The model under review builds one solid part; all positions refer to its coordinate system, in mm. A direction names the side the tool comes from. Round coordinates to 2 decimals unless told otherwise and drop trailing zeros. Loops run counter-clockwise (first coordinate to the right, second up) from the corner with the lowest first, then second, coordinate; pieces in that order, holes last. Notation, with made-up numbers: (46.25, 44) -> (67.25, 44) arc R20 cw to (67.25, 73) -> close; hole circle Ø7 at (-3, 11.25). An arc over 180 degrees is marked (long way). Use a Markdown table: item, result. Add a question column.
1) Consider section A-A on y = 3.75. Give the boundary of the cut face in (x, z).
2) Insertion check: pin 1 (1.6 mm diameter, centred on y = 5.715, z = -11.525, fed in from +X); pin 2 (4 mm diameter, centred on x = 8.5, y = 6.5, fed in from -Z). Each pin has a flat end and moves straight along its axis. Give the tip position at first contact, or say it passes through.
3) Wall thickness on probe 1 along X at (y, z) = (6, -9.5); probe 2 along Y at (x, z) = (1.25, -20.5) (3 decimals); probe 3 along Z at (x, y) = (5.75, 5.75): over which ranges is each line inside the solid? List them lowest first.
4) For faces 1 (the flat face through (-11.112, 2, -2)), 2 (the flat face through (8, 6, -14.7)), 3 (the flat face through (-8, 6, -8.35)), 4 (the flat face through (-4.762, 4, -11)), 5 (the flat face through (0, 2, 20.6)), list the 3-axis set-ups (+Z, -Z, +X, -X, +Y, -Y) from which the entire face can be reached by the end or side of a thin tool; tool diameter is ignored.
5) Consider section C-C on z = -4. Give the boundary of the cut face in (x, y) (1 decimal).
6) Mouldability with a two-part tool opening along Y and no side actions: class faces 6 (the flat face through (4.762, 4, -11)), 7 (the flat face through (8, 7.984, -12)), 8 (the cylindrical face through (7.982, 4.826, -11.988)), 9 (the flat face through (0, 0, -3)) as released by +Y, released by -Y, zero draft, split by the parting line, or undercut.
from build123d import *

# Parameters (mm, degrees)
SKETCH1_W             = 22.225
SKETCH1_H             = 46
BOSS_EXTRUDE1_DEPTH   = 3.175
SKETCH2_W             = 6.35
SKETCH2_H             = 6.35
BOSS_EXTRUDE2_DEPTH   = 4.80949
F_1_0MM_DOWEL_HOLE1_D = 2.005


with BuildPart() as part:
    # Sketch1 → Boss-Extrude1 (new body)
    with BuildSketch(Plane(origin=(0, 0, 0), x_dir=(1, 0, 0), z_dir=(0, 1, 0))):
        with Locations((0, 2.4)):
            Rectangle(SKETCH1_W, SKETCH1_H)
    extrude(amount=BOSS_EXTRUDE1_DEPTH)

    # Sketch2 → Boss-Extrude2 (add)
    with BuildSketch(Plane(origin=(0, 3.175, 0), x_dir=(1, 0, 0), z_dir=(0, 1, 0))):
        with Locations((7.9375, 11.525)):
            Rectangle(SKETCH2_W, SKETCH2_H)
    boss_extrude2 = extrude(amount=BOSS_EXTRUDE2_DEPTH)

    # Ø1.0mm Dowel Hole1 (through all)
    with Locations(Plane.ZY.offset(-4.7625)):
        with Locations((-11.525, 5.715)):
            f_1_0mm_dowel_hole1 = Hole(F_1_0MM_DOWEL_HOLE1_D / 2)

    # Mirror1: Boss-Extrude2, Ø1.0mm Dowel Hole1 across plane
    add(boss_extrude2.mirror(Plane.ZY))
    add(f_1_0mm_dowel_hole1.mirror(Plane.ZY), mode=Mode.SUBTRACT)


solid = part.part
Result set:
| question | item | result |
|---|---|---|
| 1 | outline | (-11.11, -14.7) -> (-4.76, -14.7) -> (-4.76, -8.35) -> (-11.11, -8.35) -> close; (4.76, -14.7) -> (11.11, -14.7) -> (11.11, -8.35) -> (4.76, -8.35) -> close |
| 2 | pin 1 | through |
| 2 | pin 2 | z = -14.7 |
| 3 | probe 1 | -11.11 to -4.76, 4.76 to 11.11 |
| 3 | probe 2 | 0 to 3.175 |
| 3 | probe 3 | -14.7 to -12.53, -10.52 to -8.35 |
| 4 | face 1 | +Z, -Z, -X, +Y, -Y |
| 4 | face 2 | -Z, +X, -X, +Y |
| 4 | face 3 | +Z, +X, -X, +Y |
| 4 | face 4 | +Z, -Z, +Y |
| 4 | face 5 | +Z, +X, -X, +Y, -Y |
| 5 | outline | (-11.1, 0) -> (11.1, 0) -> (11.1, 3.2) -> (-11.1, 3.2) -> close |
| 6 | face 6 | zero draft |
| 6 | face 7 | released by +Y |
| 6 | face 8 | undercut |
| 6 | face 9 | released by -Y |
